Build history of the part. All positions in model axes, mm. Face numbers are marked on the shaded views. A direction names the side the tool comes from. Give positions to 0.01 mm unless a question says otherwise; leave off trailing zeros. Order: outer loops, then holes, each group sorted by start corner. A loop starts at its lowest first (then second) coordinate and runs counter-clockwise, first axis right, second up. Notation, with made-up numbers: M 11,-14.75 L 25,-14.75 A35 ccw 25,19.25 Z; hole C 44,-16 d10. An arc over 180 degrees is marked long. One line per item, written item: value.
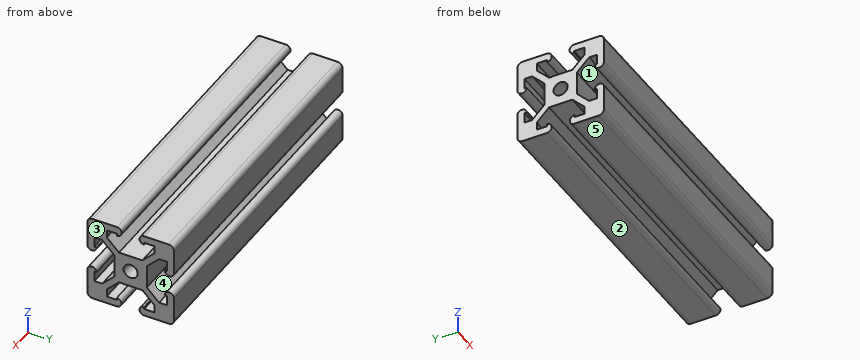
from build123d import *

# Parameters (mm, degrees)
SKETCH1_R           = 3.25
BOSS_EXTRUDE1_DEPTH = 140


with BuildPart() as part:
    # Sketch1 → Boss-Extrude1 (new body)
    with BuildSketch(Plane(origin=(0, 0, 0), x_dir=(0, 0, -1), z_dir=(1, 0, 0))):
        with BuildLine():
            Line((-20, 17.5), (-20, 6.25))
            ThreePointArc((-20, 6.25), (-17.85, 4.1), (-15.7, 6.25))
            Line((-15.7, 6.25), (-16.7, 6.25))
            Line((-16.7, 6.25), (-16.7, 11.005533085))
            Line((-16.7, 11.005533085), (-13.126853428, 11.005533085))
            Line((-13.126853428, 11.005533085), (-7.5, 5.378679656))
            Line((-7.5, 5.378679656), (-7.5, -5.378679656))
            Line((-7.5, -5.378679656), (-13.126853428, -11.005533085))
            Line((-13.126853428, -11.005533085), (-16.7, -11.005533085))
            Line((-16.7, -11.005533085), (-16.7, -6.25))
            Line((-16.7, -6.25), (-15.7, -6.25))
            ThreePointArc((-15.7, -6.25), (-17.85, -4.1), (-20, -6.25))
            Line((-20, -6.25), (-20, -17.5))
            ThreePointArc((-20, -17.5), (-19.267766953, -19.267766953), (-17.5, -20))
            Line((-17.5, -20), (-6.25, -20))
            ThreePointArc((-6.25, -20), (-4.1, -17.85), (-6.25, -15.7))
            Line((-6.25, -15.7), (-6.25, -16.7))
            Line((-6.25, -16.7), (-11.005533085, -16.7))
            Line((-11.005533085, -16.7), (-11.005533085, -13.126853428))
            Line((-11.005533085, -13.126853428), (-5.378679656, -7.5))
            Line((-5.378679656, -7.5), (5.378679656, -7.5))
            Line((5.378679656, -7.5), (11.005533085, -13.126853428))
            Line((11.005533085, -13.126853428), (11.005533085, -16.7))
            Line((11.005533085, -16.7), (6.25, -16.7))
            Line((6.25, -16.7), (6.25, -15.7))
            ThreePointArc((6.25, -15.7), (4.1, -17.85), (6.25, -20))
            Line((6.25, -20), (17.5, -20))
            ThreePointArc((17.5, -20), (19.267766953, -19.267766953), (20, -17.5))
            Line((20, -17.5), (20, -6.376005661))
            ThreePointArc((20, -6.376005661), (17.85, -4.226005661), (15.7, -6.376005661))
            Line((15.7, -6.376005661), (16.7, -6.376005661))
            Line((16.7, -6.376005661), (16.7, -11.005533085))
            Line((16.7, -11.005533085), (13.126853428, -11.005533085))
            Line((13.126853428, -11.005533085), (7.5, -5.378679656))
            Line((7.5, -5.378679656), (7.5, 5.378679656))
            Line((7.5, 5.378679656), (13.126853428, 11.005533085))
            Line((13.126853428, 11.005533085), (16.7, 11.005533085))
            Line((16.7, 11.005533085), (16.7, 6.25))
            Line((16.7, 6.25), (15.7, 6.25))
            ThreePointArc((15.7, 6.25), (17.85, 4.1), (20, 6.25))
            Line((20, 6.25), (20, 17.5))
            ThreePointArc((20, 17.5), (19.267766953, 19.267766953), (17.5, 20))
            Line((17.5, 20), (6.25, 20))
            ThreePointArc((6.25, 20), (4.1, 17.85), (6.25, 15.7))
            Line((6.25, 15.7), (6.25, 16.7))
            Line((6.25, 16.7), (11.005533085, 16.7))
            Line((11.005533085, 16.7), (11.005533085, 13.126853428))
            Line((11.005533085, 13.126853428), (5.378679656, 7.5))
            Line((5.378679656, 7.5), (-5.378679656, 7.5))
            Line((-5.378679656, 7.5), (-11.005533085, 13.126853428))
            Line((-11.005533085, 13.126853428), (-11.005533085, 16.7))
            Line((-11.005533085, 16.7), (-6.25, 16.7))
            Line((-6.25, 16.7), (-6.25, 15.7))
            ThreePointArc((-6.25, 15.7), (-4.1, 17.85), (-6.25, 20))
            Line((-6.25, 20), (-17.5, 20))
            ThreePointArc((-17.5, 20), (-19.267766953, 19.267766953), (-20, 17.5))
        make_face()
        Circle(SKETCH1_R, mode=Mode.SUBTRACT)
    extrude(amount=BOSS_EXTRUDE1_DEPTH)


solid = part.part
1) Mould opens along Z. For the marked faces 3, 4 and 5 say: released by +Z, released by -Z, zero draft, split by the parting line, or undercut.
Check values:
face 3: zero draft
face 4: undercut
face 5: released by -Z
2) Saw through at A-A, the plane y = 0. Write the cut outline in (x, z), then the cut area to 3 significant figures.
Check values:
outline: M 0,-7.5 L 140,-7.5 L 140,-3.25 L 0,-3.25 Z; M 0,3.25 L 140,3.25 L 140,7.5 L 0,7.5 Z
area: 1,190 mm^2
3) Drill centre lines: probe 1 along Y at (x, z) = (74.5, -14); probe 2 along Z at (x, y) = (31.5, -6); probe 3 along Y at (x, z) = (94.5, -17.5). Where is each one in solid material? Low to high. Write a range as from..to.
Check values:
probe 1: -20..-11.01, 11.01..20
probe 2: -19.97..-15.73, -8.12..8.12, 15.71..19.99
probe 3: -20..-4.25, 4.13..20
4) Tool access for the marked faces 1 and 2: list every direction of +Z, -Z, +X, -X, +Y, -Y with a clear straight run to the whole face (end or side of a thin tool).
Check values:
face 1: +X, -X
face 2: -Z, +X, -X, +Y, -Y
5) Pin check, flat tips, straight feed: pin 1 (8.5 mm diameter, centred on x = 94, z = -1, fed in from +Y); pin 2 (6 mm diameter, centred on y = 0, z = 0, fed in from -X); pin 3 (3 mm diameter, centred on x = 95, z = -2, fed in from -Y); pin 4 (5.5 mm diameter, centred on x = 45.5, y = 2, fed in from +Z). Stop position of each tip, or through.
Check values:
pin 1: y = 19.75
pin 2: through
pin 3: y = -7.5
pin 4: z = 19.39
